For this review, use the dimensioned drawing (mm, ordinates from the lowest corner) and the shaded views. A direction names the side the tool comes from. Round coordinates to 2 decimals unless told otherwise and drop trailing zeros. One line per item, written item: value. Start each with the question number.
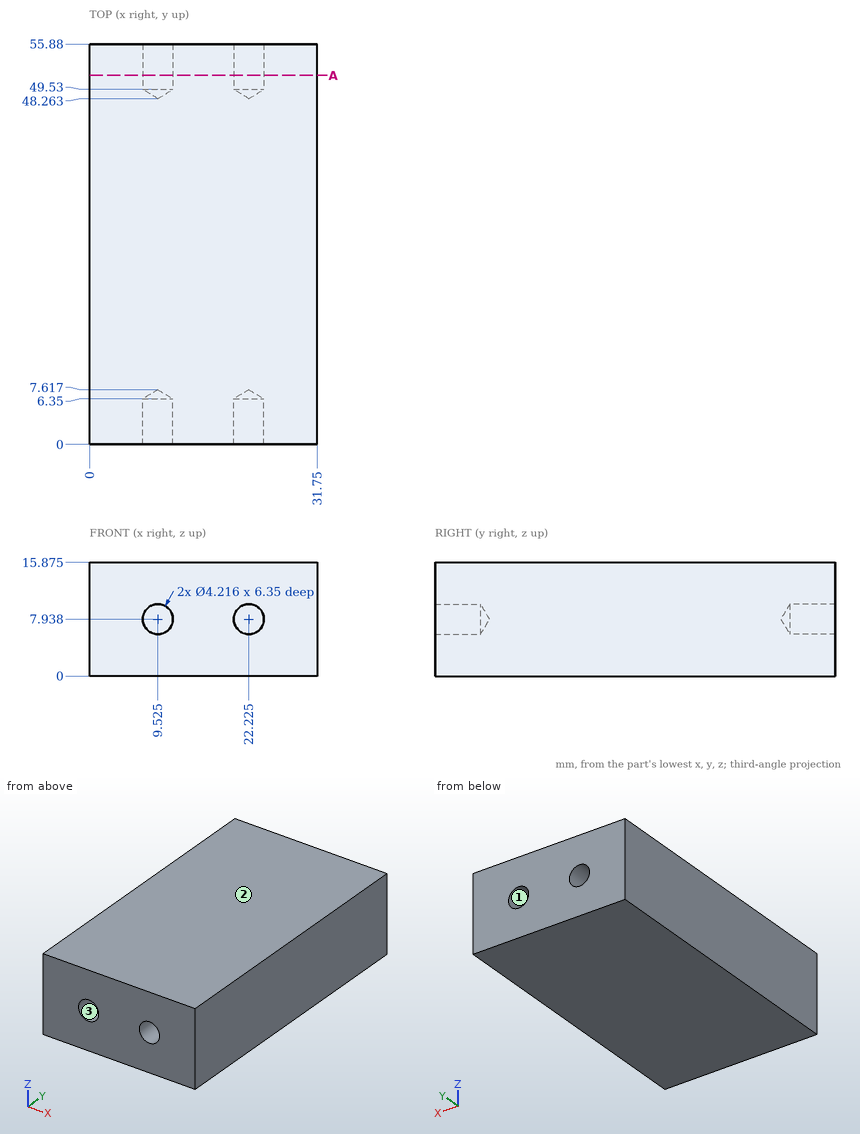
Item 1: Wall thickness on L1, parallel to Z at x = 8, y = 50 (1 decimal); L2, parallel to Y at x = 24, z = 7.75 (1 decimal): over which ranges is each line inside the solid? List them lowest first.
Item 2: Machinability: for the marked faces 1, 2 and 3, which of the approach directions +Z, -Z, +X, -X, +Y, -Y give a long, thin tool a straight path to every point of the face, cutting with its end or side? Answer none if there is none.
Item 3: Consider section A-A, the plane y = 51.5. Count the separate pieces of the cut face and the enclosed holes in it, then the cut area to 3 significant figures.
Item 4: Clearance check with flat-ended pins moving along their axes: P1, Ø2.5, axis at x = 22.22, z = 7.94, coming from the +Y side; P2, Ø4, axis at x = 9.52, z = 7.94, coming from the -Y side; P3, Ø3.5, axis at x = 9.52, z = 7.94, coming from the -Y side. State where each tip first meets the part, or that it passes through.
Computed:
1. L1: z = 0 to 6.5, 9.4 to 15.9
1. L2: y = 6.5 to 49.3
2. face 1: +Y
2. face 2: +Z, +X, -X, +Y, -Y
2. face 3: -Y
3. separate pieces: 1
3. enclosed holes: 2
3. area: 476 mm^2
4. P1: stops at y = 49.02
4. P2: stops at y = 6.41
4. P3: stops at y = 6.56
